For this review, take the finished solid that the model builds, in its own axes (mm). A direction names the side the tool comes from. Round coordinates to 2 decimals unless told otherwise and drop trailing zeros. Write each loop counter-clockwise with the first axis right and the second up, starting at its lowest first coordinate (ties: lowest second). Pieces come first, ordered by that corner, then holes. Notation, with made-up numbers: (0, -30) -> (15, -30) arc R28 ccw to (15, -12) -> close; hole circle Ø6 at (-13.75, 50.25). An arc over 180 degrees is marked (long way). Write item = value, one per line. Start each with the question number.
```python
from build123d import *

# Parameters (mm, degrees)
BOSS_EXTRUDE1_DEPTH                     = 27
CBORE_FOR_M5_HEX_HEAD_BOLT1_D           = 30
CBORE_FOR_M5_HEX_HEAD_BOLT1_CBORE_D     = 38
CBORE_FOR_M5_HEX_HEAD_BOLT1_CBORE_DEPTH = 4
SKETCH5_W                               = 13
SKETCH5_H                               = 53.5
CUT_EXTRUDE2_DEPTH                      = 140.582412932
CUT_EXTRUDE3_DEPTH                      = 140.582412932
CUT_EXTRUDE3_DEPTH_BACK                 = 140.582412932
CUT_EXTRUDE4_DEPTH                      = 141.36470354
FILLET1_R                               = 6
FILLET2_R                               = 6


with BuildPart() as part:
    # Sketch1 → Boss-Extrude1 (new body)
    with BuildSketch(Plane.YZ):
        with BuildLine():
            Line((0, 0), (0, 42))
            ThreePointArc((0, 42), (27.5, 69.5), (55, 42))
            Line((55, 42), (55, 28))
            ThreePointArc((55, 28), (58.514718626, 19.514718626), (67, 16))
            Line((67, 16), (118, 16))
            Line((118, 16), (118, 0))
            Line((118, 0), (0, 0))
        make_face()
    extrude(amount=-BOSS_EXTRUDE1_DEPTH)

    # CBORE for M5 Hex Head Bolt1 (through all)
    with Locations(Plane.YZ):
        with Locations((27.5, 42)):
            CounterBoreHole(CBORE_FOR_M5_HEX_HEAD_BOLT1_D / 2, CBORE_FOR_M5_HEX_HEAD_BOLT1_CBORE_D / 2, CBORE_FOR_M5_HEX_HEAD_BOLT1_CBORE_DEPTH)

    # Sketch5 → Cut-Extrude2 (cut, through all)
    with BuildSketch(Plane.XZ):
        with Locations((-20.5, 42.75)):
            Rectangle(SKETCH5_W, SKETCH5_H)
    extrude(amount=-CUT_EXTRUDE2_DEPTH, mode=Mode.SUBTRACT)

    # Sketch6 → Cut-Extrude3 (cut, two sides: drawn at the far end of the back side and taken through both)
    with BuildSketch(Plane.XZ.offset(-CUT_EXTRUDE3_DEPTH_BACK)):
        Polygon((-92.317950055, -132.186567024), (-16, 0), (-11.381197846, 8), (-27, 8), (-179.635900109, 8), (-438.753666214, -153.396577713), (-351.43571616, -293.583144737), align=None)
    extrude(amount=CUT_EXTRUDE3_DEPTH + CUT_EXTRUDE3_DEPTH_BACK, mode=Mode.SUBTRACT)

    # Mirror1: part across plane


with BuildPart() as part_1:
    add(part.part)
    add(part.part.mirror(Plane(origin=(-27, 27.5, 42), x_dir=(0, 0, 1), z_dir=(-1, 0, 0))))

    # Sketch7 → Cut-Extrude4 (cut, through all)
    with BuildSketch(Plane.XY.offset(16)):
        with BuildLine():
            Line((-19, 101), (-19, 18))
            ThreePointArc((-19, 18), (-27, 10), (-35, 18))
            Line((-35, 18), (-35, 101))
            ThreePointArc((-35, 101), (-27, 109), (-19, 101))
        make_face()
    extrude(amount=-CUT_EXTRUDE4_DEPTH, mode=Mode.SUBTRACT)

    # Fillet1
    # the kernel refuses this fillet: 6 mm, written as the material it takes off along each edge
    with BuildSketch(Plane(origin=(0, 0, -36), x_dir=(0, 1, 0), z_dir=(0, 0, 1))) as fillet1_piece_1:
        with BuildLine():
            CenterArc((FILLET1_R, FILLET1_R), FILLET1_R, 180, 90)
            Line((0, FILLET1_R), (-FILLET1_R * 0.02, FILLET1_R))
            Line((-FILLET1_R * 0.02, FILLET1_R), (-FILLET1_R * 0.02, -FILLET1_R * 0.02))
            Line((-FILLET1_R * 0.02, -FILLET1_R * 0.02), (FILLET1_R, -FILLET1_R * 0.02))
            Line((FILLET1_R, -FILLET1_R * 0.02), (FILLET1_R, 0))
        make_face()
    extrude(amount=114, mode=Mode.SUBTRACT)

    # Fillet2
    # the kernel refuses this fillet: 6 mm, written as the material it takes off along each edge
    with BuildSketch(Plane(origin=(-54, 0, -36), x_dir=(0, 1, 0), z_dir=(0, 0, 1))) as fillet2_piece_1:
        with BuildLine():
            CenterArc((FILLET2_R, -FILLET2_R), FILLET2_R, 90, 90)
            Line((0, -FILLET2_R), (-FILLET2_R * 0.02, -FILLET2_R))
            Line((-FILLET2_R * 0.02, -FILLET2_R), (-FILLET2_R * 0.02, FILLET2_R * 0.02))
            Line((-FILLET2_R * 0.02, FILLET2_R * 0.02), (FILLET2_R, FILLET2_R * 0.02))
            Line((FILLET2_R, FILLET2_R * 0.02), (FILLET2_R, 0))
        make_face()
    extrude(amount=114, mode=Mode.SUBTRACT)
    with BuildSketch(Plane(origin=(-54, 118, 52), x_dir=(1, 0, 0), z_dir=(0, 0, -1)), Plane(origin=(0, 118, 52), x_dir=(0, -1, 0), z_dir=(0, 0, -1))) as fillet2_piece_2:
        with BuildLine():
            CenterArc((FILLET2_R, FILLET2_R), FILLET2_R, 180, 90)
            Line((0, FILLET2_R), (-FILLET2_R * 0.02, FILLET2_R))
            Line((-FILLET2_R * 0.02, FILLET2_R), (-FILLET2_R * 0.02, -FILLET2_R * 0.02))
            Line((-FILLET2_R * 0.02, -FILLET2_R * 0.02), (FILLET2_R, -FILLET2_R * 0.02))
            Line((FILLET2_R, -FILLET2_R * 0.02), (FILLET2_R, 0))
        make_face()
    extrude(amount=88, mode=Mode.SUBTRACT)


solid = part_1.part
```
1. Machinability: for faces 5 (the flat face through (-4, 13, 36)), 6 (the flat face through (-14, 26, 25)), 7 (the flat face through (-35, 59, 12)), 8 (the flat face through (-7, 55, 35)), which of the approach directions +Z, -Z, +X, -X, +Y, -Y give a long, thin tool a straight path to every point of the face, cutting with its end or side? Answer none if there is none.
2. Consider section A-A, the plane y = 27.5. Give the number of separate pieces and of enclosed holes in the cut face, then the cut area to 3 significant figures.
3. Consider section B-B, the plane x = -8.5. Give the boundary of the cut face in (y, z), then the cut area to 3 significant figures.
4. Wall thickness on L1, parallel to Z at x = -1, y = 27; L2, parallel to X at y = 53, z = 36; L3, parallel to Z at x = -7, y = 27.5: over which ranges is each line inside the solid? List them lowest first. Write a range as from..to.
5. Consider section C-C, the plane x = -27. Give the boundary of the cut face in (y, z).
6. Draft analysis for pull direction Z (two halves, no side actions). For faces 1 (the cylindrical face through (-6.9, 58.42, 19.61)), 2 (the flat face through (-8, 60, 0)), 3 (the flat face through (-38, 60, 8)), 4 (the cylindrical face through (-52.289, 1.804, 29.159)), state which applies: +Z half, -Z half, draft (parallel to the pull), parting line (faces both ways), or undercut.
7. Clearance check with flat-ended pins moving along their axes: pin 1 Ø10 at (x, y) = (-8.5, 76.5) entering from +Z; pin 2 Ø4 at (x, z) = (-8.5, 36) entering from +Y; pin 3 Ø1 at (x, z) = (-44.5, 59) entering from +Y. State where each tip first meets the part, or that it passes through.
8. Consider section D-D, the plane x = -20.5. Give the boundary of the cut face in (y, z).
Outcome:
q1.face_5 = +X
q1.face_6 = +Z, +Y, -Y
q1.face_7 = +Z, -Z
q1.face_8 = +Z, +X, -X, +Y
q2.separate_pieces = 4
q2.enclosed_holes = 0
q2.area = 1,120 mm2
q3.outline = (0, 0) -> (118, 0) -> (118, 16) -> (67, 16) arc R12 cw to (55, 28) -> (55, 42) arc R27.5 ccw to (0, 42) -> close; hole circle Ø30 at (27.5, 42)
q3.area = 3,830 mm2
q4.L1 = 0..23.01, 60.99..69.5
q4.L2 = -54..-40, -14..0
q4.L3 = 0..27, 57..69.5
q5.outline = (0, 8) -> (10, 8) -> (10, 16) -> (0, 16) -> close; (109, 8) -> (118, 8) -> (118, 16) -> (109, 16) -> close
q6.face_1 = +Z half
q6.face_2 = -Z half
q6.face_3 = undercut
q6.face_4 = draft
q7.pin_1 = 16
q7.pin_2 = 55
q7.pin_3 = 49.5
q8.outline = (0, 8) -> (13.34, 8) -> (13.34, 16) -> (0, 16) -> close; (105.66, 8) -> (118, 8) -> (118, 16) -> (105.66, 16) -> close
